```python
from build123d import *

# Parameters (mm, degrees)
CROQUIS1_W              = 18
CROQUIS1_H              = 18
CROQUIS1_R              = 1.55
SALIENTE_EXTRUIR1_DEPTH = 3
CROQUIS3_W              = 18
CROQUIS3_H              = 10
SALIENTE_EXTRUIR3_DEPTH = 3
CORTAR_EXTRUIR1_REACH   = 28.153
CROQUIS4_W              = 2
CROQUIS4_H              = 10
CROQUIS14_W             = 16
CROQUIS14_H             = 10
SALIENTE_EXTRUIR8_DEPTH = 9
CORTAR_EXTRUIR2_DEPTH   = 3
REDONDEO1_R             = 1


with BuildPart() as part:
    # Croquis1 → Saliente-Extruir1 (new body)
    with BuildSketch(Plane(origin=(0, 0, 0), x_dir=(1, 0, 0), z_dir=(0, 1, 0))):
        with Locations((9, 9)):
            Rectangle(CROQUIS1_W, CROQUIS1_H)
        with Locations(Location((3.5, 3, 0), (0, 0, 270))):
            Circle(CROQUIS1_R, mode=Mode.SUBTRACT)
    extrude(amount=SALIENTE_EXTRUIR1_DEPTH)

    # Croquis3 → Saliente-Extruir3 (add)
    with BuildSketch(Plane(origin=(0, 3, 0), x_dir=(1, 0, 0), z_dir=(0, 1, 0))):
        with Locations((9, 13)):
            Rectangle(CROQUIS3_W, CROQUIS3_H)
    extrude(amount=SALIENTE_EXTRUIR3_DEPTH)

    # Cortar-Extruir1: up to this face of the body (flat: up to its plane)
    cortar_extruir1_end = Plane(part.part.faces().sort_by_distance((9, 6, -13))[0])
    # Croquis4 → Cortar-Extruir1 (cut, up to the picked face)
    with BuildSketch(Plane.XZ, mode=Mode.PRIVATE) as cortar_extruir1_sk1:
        with Locations((1, -13)):
            Rectangle(CROQUIS4_W, CROQUIS4_H)
    cortar_extruir1_tool1 = split(extrude(cortar_extruir1_sk1.sketch, amount=-CORTAR_EXTRUIR1_REACH, mode=Mode.PRIVATE), bisect_by=cortar_extruir1_end, keep=Keep.BOTH, mode=Mode.PRIVATE)
    add(cortar_extruir1_tool1.solids().sort_by(Axis((1, 0, -13), (0, 1, 0)))[0], mode=Mode.SUBTRACT)

    # Croquis14 → Saliente-Extruir8 (add)
    with BuildSketch(Plane(origin=(0, 6, 0), x_dir=(1, 0, 0), z_dir=(0, 1, 0))):
        with Locations((10, 13)):
            Rectangle(CROQUIS14_W, CROQUIS14_H)
    extrude(amount=SALIENTE_EXTRUIR8_DEPTH)

    # Croquis15 → Cortar-Extruir2 (cut)
    with BuildSketch(Plane(origin=(18, 0, 0), x_dir=(0, 0, -1), z_dir=(1, 0, 0))):
        Polygon((0, 0), (18, 0), (18, 15), (8, 15), (8, 3), (0, 3), align=None)
    extrude(amount=-CORTAR_EXTRUIR2_DEPTH, mode=Mode.SUBTRACT)

    # Redondeo1
    redondeo1_edges = [part.edges().sort_by_distance(p)[0] for p in [
        (0, 1.5, -8),
        (2, 7.5, -18),
        (2, 9, -8),
        (15, 1.5, 0),
        (15, 9, -8),
        (15, 7.5, -18),
        (0, 1.5, 0),
    ]]
    fillet(redondeo1_edges, radius=REDONDEO1_R)


solid = part.part
```
Work out the finished part from the listing and answer in its coordinate system (mm). A direction names the side the tool comes from. Give positions to 0.01 mm unless a question says otherwise; leave off trailing zeros. Write each loop counter-clockwise with the first axis right and the second up, starting at its lowest first coordinate (ties: lowest second). Pieces come first, ordered by that corner, then holes. Notation, with made-up numbers: (-23.5, 25) -> (-3.5, 25) arc R21 ccw to (-3.5, 38) -> close; hole circle Ø6 at (67, 27). An arc over 180 degrees is marked (long way). Write item = value, one per line.
Q1. Consider line 1 along X through (y, z) = (1.3, -3); line 2 along X through (y, z) = (2.25, -12.25); line 3 along Y through (x, z) = (3.75, -7.75). Determine where each line is inside the solid, lowest interval first.
Computed values:
line_1 = 0 to 1.95, 5.05 to 15
line_2 = 2 to 15
line_3 = 0 to 3
Q2. Section A-A on x = 3.5 is taken. Determine the outline of the cut face in (y, z), and give its area (3 significant figures).
Computed values:
outline = (0, -18) -> (15, -18) -> (15, -8) -> (3, -8) -> (3, -4.55) -> (0, -4.55) -> close; (0, -1.45) -> (3, -1.45) -> (3, 0) -> (0, 0) -> close
area = 165 mm^2
Q3. Flat-ended cylindrical pins translate along their axes: pin 1 Ø2.5 at (y, z) = (10, -12) entering from -X; pin 2 Ø8 at (x, y) = (10.5, 10) entering from +Z. Find the tip coordinate at first contact, or state that the pin passes through.
Computed values:
pin_1 = 2
pin_2 = -8
Q4. A tool of negligible diameter and unlimited length cuts with its end or side. For faces 1 (the flat face through (2, 7, -12)), 2 (the flat face through (8, 9, -8)), 3 (the cylindrical face through (2.285, 9.084, -8.301)), 4 (the cylindrical face through (14.699, 8.916, -8.285)), from which of +Z, -Z, +X, -X, +Y, -Y can it reach the whole face along a straight path? Write none if from no direction.
Computed values:
face_1 = -Z, -X, +Y, -Y
face_2 = +Z, +X, -X, +Y
face_3 = +Z, -X, +Y
face_4 = +Z, +X, +Y
Q5. Section B-B on z = -3 is taken. Determine the outline of the cut face in (x, y), and give its area (3 significant figures).
Computed values:
outline = (0, 0) -> (1.95, 0) -> (1.95, 3) -> (0, 3) -> close; (5.05, 0) -> (15, 0) -> (15, 3) -> (5.05, 3) -> close
area = 35.7 mm^2
Q6. Section C-C on y = 2.25 is taken. Determine the outline of the cut face in (x, z), and give its area (3 significant figures).
Computed values:
outline = (0, -7) arc R1 ccw to (1, -8) -> (2, -8) -> (2, -17) arc R1 ccw to (3, -18) -> (14, -18) arc R1 ccw to (15, -17) -> (15, -1) arc R1 ccw to (14, 0) -> (1, 0) arc R1 ccw to (0, -1) -> close; hole circle Ø3.1 at (3.5, -3)
area = 241 mm^2
Q7. Section D-D on y = 11 is taken. Determine the outline of the cut face in (x, z).
Computed values:
outline = (2, -17) arc R1 ccw to (3, -18) -> (14, -18) arc R1 ccw to (15, -17) -> (15, -9) arc R1 ccw to (14, -8) -> (3, -8) arc R1 ccw to (2, -9) -> close
